```python
from build123d import *

# Parameters (mm, degrees)
SALIENTE_EXTRUIR1_DEPTH = 10


with BuildPart() as part:
    # Croquis1 → Saliente-Extruir1 (new body)
    with BuildSketch(Plane.XY):
        with BuildLine():
            Line((-25, 9.844348503), (-25, 0))
            Line((-25, 0), (25, 0))
            Line((25, 0), (25, 9.844348503))
            Line((25, 9.844348503), (30, 9.844348503))
            Line((30, 9.844348503), (30, 0))
            Line((30, 0), (67, 0))
            Line((67, 0), (67, 17.097567982))
            Line((67, 17.097567982), (74.5, 17.097567982))
            ThreePointArc((74.5, 17.097567982), (82, 24.597567982), (74.5, 32.097567982))
            Line((74.5, 32.097567982), (67, 32.097567982))
            Line((67, 32.097567982), (67, 50))
            Line((67, 50), (-67, 50))
            Line((-67, 50), (-67, 32.097567982))
            Line((-67, 32.097567982), (-74.5, 32.097567982))
            ThreePointArc((-74.5, 32.097567982), (-82, 24.597567982), (-74.5, 17.097567982))
            Line((-74.5, 17.097567982), (-67, 17.097567982))
            Line((-67, 17.097567982), (-67, 0))
            Line((-67, 0), (-30, 0))
            Line((-30, 0), (-30, 9.844348503))
            Line((-30, 9.844348503), (-25, 9.844348503))
        make_face()
        with BuildLine():
            Line((59.5, 13.1), (-59.5, 13.1))
            Line((-59.5, 13.1), (-59.5, 17.097567982))
            Line((-59.5, 17.097567982), (-59.5, 32.097567982))
            Line((-59.5, 32.097567982), (-59.5, 36.7))
            ThreePointArc((-59.5, 36.7), (-56.571067812, 43.771067812), (-49.5, 46.7))
            Line((-49.5, 46.7), (44.1, 46.7))
            Line((44.1, 46.7), (49.5, 46.7))
            ThreePointArc((49.5, 46.7), (56.571067812, 43.771067812), (59.5, 36.7))
            Line((59.5, 36.7), (59.5, 13.1))
        make_face(mode=Mode.SUBTRACT)
    extrude(amount=SALIENTE_EXTRUIR1_DEPTH)


solid = part.part
```
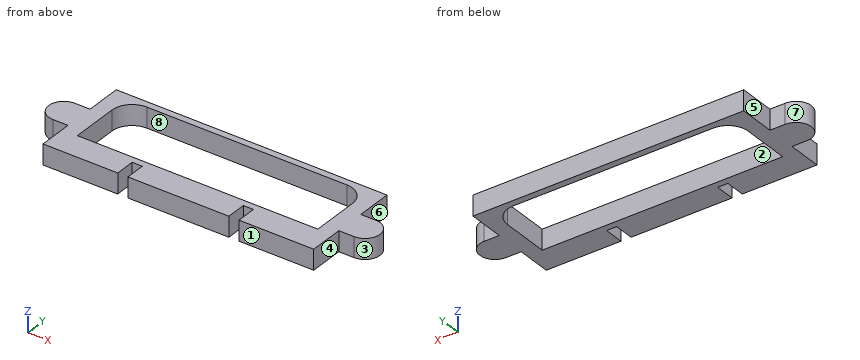
CAD build for the part. Positions are in the model's coordinates, mm. Face numbers are marked on the shaded views. A direction names the side the tool comes from. Give positions to 0.01 mm unless a question says otherwise; leave off trailing zeros. Write each loop counter-clockwise with the first axis right and the second up, starting at its lowest first coordinate (ties: lowest second). Pieces come first, ordered by that corner, then holes. Notation, with made-up numbers: M 75.5,-15.75 L 110.5,-15.75 A17 ccw 110.5,17.25 Z; hole C 54.5,-4 d6. An arc over 180 degrees is marked long. Return JSON: item names as keys, results as strings. Group by question number.
(1) Band-saw the part on C-C (z = 6.5). Give the cut face in (x, y), and give its area (3 significant figures).
(2) Mould opens along X. For the marked faces 1, 2 and 3 say: pulls with the +X half, pulls with the -X half, needs draft (parallel to the pull), parting line crosses it, or undercut.
(3) Band-saw the part on B-B (y = 3.5). Give the cut face in (x, z).
(4) Flat gauge pins, fed straight in: pin 1 Ø3 at (y, z) = (12.5, 4.5) entering from -X; pin 2 Ø1 at (y, z) = (37.5, 8.5) entering from +X; pin 3 Ø2 at (x, z) = (72, 3) entering from +Y; pin 4 Ø1 at (x, y) = (-57.5, 28.5) entering from +Z. Where does each tip first touch, or does it go through?
(5) 3-axis set-ups, long thin cutter, end or side, ignore diameter. For the marked faces 4, 5, 6, 7 and 8: which of +Z, -Z, +X, -X, +Y, -Y reach the whole face in a straight line?
(6) Drill centre lines: L1, parallel to X at y = 7.5, z = 2.25; L2, parallel to X at y = 33.5, z = 9.25; L3, parallel to Y at x = -10, z = 1. Where is each one in solid material? Low to high. Write a range as [from, to].
(7) Band-saw the part on A-A (x = -41). Give the cut face in (y, z).
(8) Band-saw the part on D-D (y = 25). Give the cut face in (x, z), and give its area (3 significant figures).
Entries:
{
 "1": {"outline": "M -74.5,17.1 L -67,17.1 L -67,0 L -30,0 L -30,9.84 L -25,9.84 L -25,0 L 25,0 L 25,9.84 L 30,9.84 L 30,0 L 67,0 L 67,17.1 L 74.5,17.1 A7.5 ccw 74.5,32.1 L 67,32.1 L 67,50 L -67,50 L -67,32.1 L -74.5,32.1 A7.5 ccw Z; hole M -59.5,13.1 L 59.5,13.1 L 59.5,36.7 A10 ccw 49.5,46.7 L -49.5,46.7 A10 ccw -59.5,36.7 Z", "area": "3,050 mm^2"},
 "2": {"face 1": "needs draft", "face 2": "undercut", "face 3": "pulls with the +X half"},
 "3": {"outline": "M -67,0 L -30,0 L -30,10 L -67,10 Z; M -25,0 L 25,0 L 25,10 L -25,10 Z; M 30,0 L 67,0 L 67,10 L 30,10 Z"},
 "4": {"pin 1": "stops at x = -67", "pin 2": "stops at x = 67", "pin 3": "stops at y = 32.1", "pin 4": "passes through"},
 "5": {"face 4": "+Z, -Z, +X, -Y", "face 5": "+Z, -Z, -X, +Y", "face 6": "+Z, -Z, +X, +Y", "face 7": "+Z, -Z, -X", "face 8": "+Z, -Z"},
 "6": {"L1": "x = [-67, -30], [-25, 25], [30, 67]", "L2": "x = [-67, -59.5], [59.5, 67]", "L3": "y = [0, 13.1], [46.7, 50]"},
 "7": {"outline": "M 0,0 L 13.1,0 L 13.1,10 L 0,10 Z; M 46.7,0 L 50,0 L 50,10 L 46.7,10 Z"},
 "8": {"outline": "M -81.99,0 L -59.5,0 L -59.5,10 L -81.99,10 Z; M 59.5,0 L 81.99,0 L 81.99,10 L 59.5,10 Z", "area": "450 mm^2"}
}
